from build123d import *

# Parameters (mm, degrees)
CUT_EXTRUDE1_START = -10
CUT_EXTRUDE1_DEPTH = 72.741396162
CIRPATTERN1_COUNT  = 4


with BuildPart() as part:
    # Sketch1 → Revolve1 (revolve)
    with BuildSketch(Plane.XY, mode=Mode.PRIVATE) as revolve1_sk:
        Polygon((11.25, 0), (11.25, 12), (19.062713823, 12), (25.848428109, 42), (32, 42), (22.5, 0), align=None)
    revolve(revolve1_sk.sketch.rotate(Axis((0, 0, 0), (0, 1, 0)), 90), axis=Axis((0, 0, 0), (0, 1, 0)))

    # Sketch2 → Cut-Extrude1 (cut)
    with BuildSketch(Plane.XY.offset(CUT_EXTRUDE1_START)):
        with BuildLine():
            Line((5, 42), (-5, 42))
            ThreePointArc((-5, 42), (0, 37), (5, 42))
        make_face()
    cut_extrude1 = extrude(amount=CUT_EXTRUDE1_DEPTH, mode=Mode.SUBTRACT)

    # CirPattern1: Cut-Extrude1 ×4 about axis
    cirpattern1_axis = Axis((0, 42, 0), (0, -1, 0))
    for i in range(1, CIRPATTERN1_COUNT):
        add(cut_extrude1.rotate(cirpattern1_axis, i * 360 / CIRPATTERN1_COUNT), mode=Mode.SUBTRACT)


solid = part.part
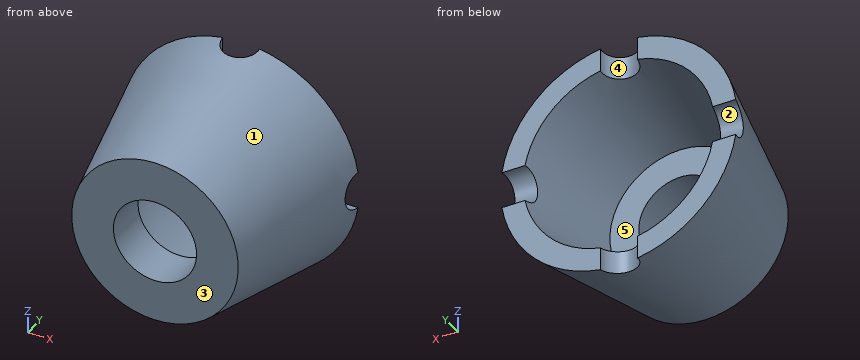
Verification items for the finished model (mm, model axes). Face numbers are marked on the shaded views. A direction names the side the tool comes from. Round coordinates to 2 decimals unless told otherwise and drop trailing zeros. Loops run counter-clockwise (first coordinate to the right, second up) from the corner with the lowest first, then second, coordinate; pieces in that order, holes last. Notation, with made-up numbers: (-17.75, 26) - (3.25, 26) arc R22 cw to (3.25, 56) - close; hole circle Ø5 at (-24.75, 64). An arc over 180 degrees is marked (long way). Write item = value, one per line.
Q1. Mould release check, pull along Z, two halves, no side actions. Record for the marked faces 1, 2 and 3: +Z half, -Z half, draft (parallel to the pull), parting line (faces both ways), or undercut.
Here are the results:
face_1 = parting line
face_2 = undercut
face_3 = draft
Q2. Sectioned sample at B-B on x = 0. Record the boundary of the cut face in (y, z).
Here are the results:
outline = (0, -22.5) - (37, -30.87) - (37, -24.72) - (12, -19.06) - (12, -11.25) - (0, -11.25) - close; (0, 11.25) - (12, 11.25) - (12, 19.06) - (37, 24.72) - (37, 30.87) - (0, 22.5) - close
Q3. Sectioned sample at D-D on y = 9. Record the boundary of the cut face in (x, z).
Here are the results:
outline = circle Ø49.07 at (0, 0); hole circle Ø22.5 at (0, 0)
Q4. Sectioned sample at C-C on y = 32.5. Record the boundary of the cut face in (x, z).
Here are the results:
outline = circle Ø59.7 at (0, 0); hole circle Ø47.4 at (0, 0)
Q5. Tool access check on the marked faces 4 and 5. Record the directions out of +Z, -Z, +X, -X, +Y, -Y that give a thin tool (end or side, any length) a straight path to the whole face; none if there is none.
Here are the results:
face_4 = +Z, -Z, +Y
face_5 = +Y
Q6. Sectioned sample at A-A on z = 0. Record the boundary of the cut face in (x, y).
Here are the results:
outline = (-30.87, 37) - (-22.5, 0) - (-11.25, 0) - (-11.25, 12) - (-19.06, 12) - (-24.72, 37) - close; (11.25, 0) - (22.5, 0) - (30.87, 37) - (24.72, 37) - (19.06, 12) - (11.25, 12) - close
Q7. Depth check by flat-ended pin: pin 1 (10 mm diameter, centred on y = 24.5, z = 16.5, fed in from -X); pin 2 (1 mm diameter, centred on x = -4, y = 5, fed in from +Z); pin 3 (4 mm diameter, centred on x = -6, y = 7, fed in from -Z); pin 4 (18 mm diameter, centred on x = 0, z = 0, fed in from -Y). Enter the tip coordinate at first touch or a pass-through.
Here are the results:
pin_1 = -25.89
pin_2 = 23.43
pin_3 = -23.97
pin_4 = through
Q8. Material ranges on L1, parallel to Y at x = 3, z = 11; L2, parallel to Z at x = 13.5, y = 22; L3, parallel to X at y = 17, z = 16, recorded low to high.
Here are the results:
L1 = 0 to 12
L2 = -23.93 to -16.51, 16.51 to 23.93
L3 = -20.93 to -12.32, 12.32 to 20.93
